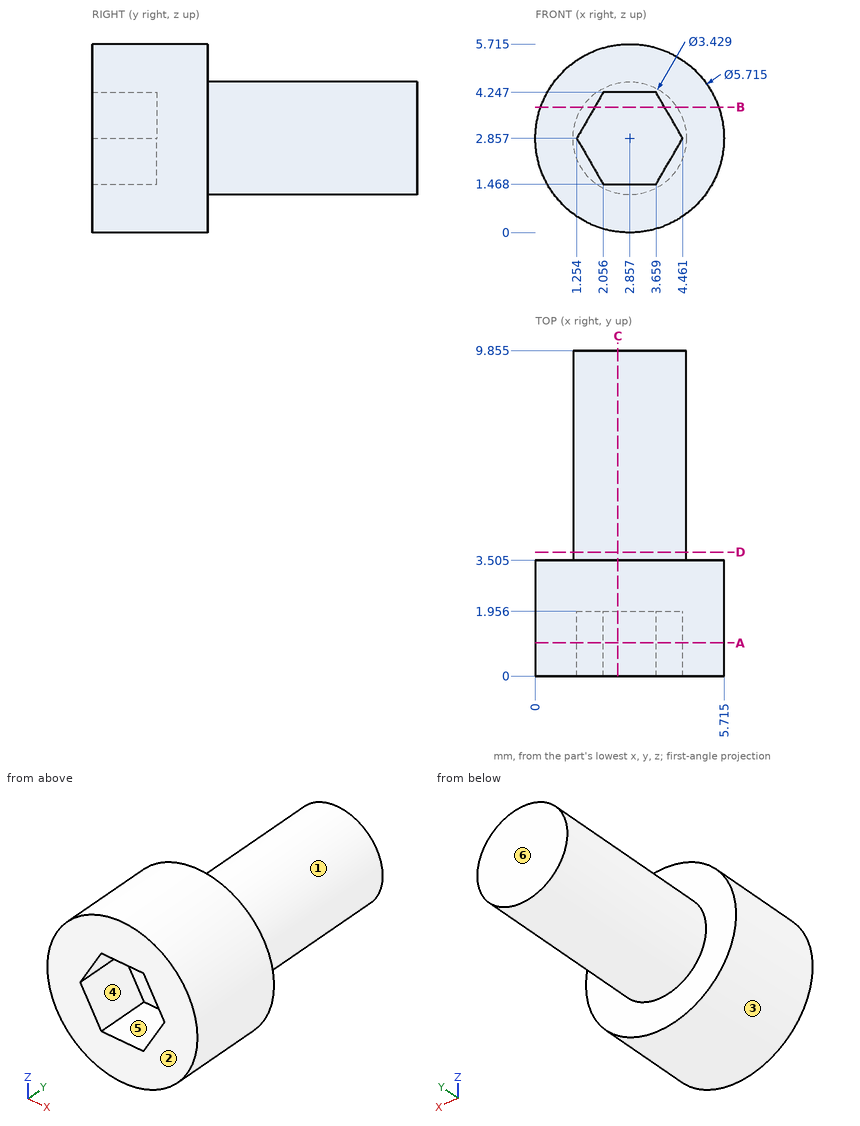
Geometry check sheet. Reference: drawing and pictorial views, mm from the part's lowest x, y, z. A direction names the side the tool comes from. Give positions to 0.01 mm unless a question says otherwise; leave off trailing zeros. Loops run counter-clockwise (first coordinate to the right, second up) from the corner with the lowest first, then second, coordinate; pieces in that order, holes last.
1. Thickness scan on line 1 (Y direction, x = 0.95, z = 3) (1 decimal); line 2 (X direction, y = 6, z = 2.75); line 3 (Y direction, x = 4.2, z = 2.7) (1 decimal). Record the ranges inside material, lowest first.
2. Section check D-D, the plane y = 3.75. Enter the section's corners in (x, z) (1 decimal).
3. Set-up check for the marked faces 1 and 2: record each of +Z, -Z, +X, -X, +Y, -Y from which the full face is reachable in a straight line by a thin tool's end or side.
4. Section check C-C, the plane x = 2.5. Enter the section's corners in (y, z) (1 decimal).
5. Go/stop test with flat-tipped pins: pin 1 Ø1 at (y, z) = (8, 4) entering from -X; pin 2 Ø1.5 at (x, z) = (3, 1) entering from +Y (1 decimal); pin 3 Ø1.5 at (x, y) = (4.5, 4) entering from -Z; pin 4 Ø0.8 at (x, z) = (3, 2.5) entering from -Y. Record where each tip stops, or that it passes through.
6. Mould release check, pull along X, two halves, no side actions. Record for the marked faces 3, 4, 5 and 6: released by +X, released by -X, zero draft, split by the parting line, or undercut.
7. Section check A-A, the plane y = 1. Enter the section's corners in (x, z) (1 decimal).
8. Section check B-B, the plane z = 3.8. Enter the section's corners in (x, y) (1 decimal).
Geometry says:
1. line 1: y = 0 to 3.5
1. line 2: x = 1.15 to 4.57
1. line 3: y = 2 to 9.9
2. outline: circle Ø3.4 at (2.9, 2.9)
3. face 1: +Y
3. face 2: +Z, -Z, +X, -X, -Y
4. outline: (0, 0) - (3.5, 0) - (3.5, 1.2) - (9.9, 1.2) - (9.9, 4.5) - (3.5, 4.5) - (3.5, 5.7) - (0, 5.7) - (0, 4.2) - (2, 4.2) - (2, 1.5) - (0, 1.5) - close
5. pin 1: stops at x = 1.27
5. pin 2: stops at y = 9.9
5. pin 3: stops at z = 0.21
5. pin 4: stops at y = 1.96
6. face 3: split by the parting line
6. face 4: undercut
6. face 5: undercut
6. face 6: zero draft
7. outline: circle Ø5.7 at (2.9, 2.9); hole (1.3, 2.9) - (2.1, 1.5) - (3.7, 1.5) - (4.5, 2.9) - (3.7, 4.2) - (2.1, 4.2) - close
8. outline: (0.2, 0) - (1.8, 0) - (1.8, 2) - (3.9, 2) - (3.9, 0) - (5.6, 0) - (5.6, 3.5) - (4.3, 3.5) - (4.3, 9.9) - (1.4, 9.9) - (1.4, 3.5) - (0.2, 3.5) - close
